CAD build for the part. Positions are in the model's coordinates, mm. Face numbers are marked on the shaded views. A direction names the side the tool comes from. Give positions to 0.01 mm unless a question says otherwise; leave off trailing zeros. Loops run counter-clockwise (first coordinate to the right, second up) from the corner with the lowest first, then second, coordinate; pieces in that order, holes last. Notation, with made-up numbers: M 80,56 L 121,56 A25 ccw 121,84 Z; hole C -0.75,9 d10. An arc over 180 degrees is marked long. Answer as CSV lines item,"result".
```python
from build123d import *

# Parameters (mm, degrees)
F0_R     = 26.67
F1_DEPTH = 3.175
F3_DEPTH = 25.4
F4_R     = 7.239
F5_DEPTH = 7.62
F7_DEPTH = 6.35
F8_R     = 2.159
F9_DEPTH = 25.4


with BuildPart() as f1:
    # F0 (on Front) → F1 (new body)
    with BuildSketch(Plane.XZ):
        Circle(F0_R)
    extrude(amount=F1_DEPTH)

    # F2 (on face) → F3 (cut)
    with BuildSketch(Plane.XZ.offset(3.175)):
        with BuildLine():
            Line((-21.59, 5.08), (-5.08, 5.08))
            Line((-5.08, 5.08), (-5.08, 21.59))
            ThreePointArc((-5.08, 21.59), (-5.221742, 22.173039), (-5.61533, 22.625934))
            ThreePointArc((-5.61533, 22.625934), (-16.90841, 16.90841), (-22.625934, 5.61533))
            ThreePointArc((-22.625934, 5.61533), (-22.173039, 5.221742), (-21.59, 5.08))
        make_face()
        with BuildLine():
            ThreePointArc((-21.59, -5.08), (-22.173039, -5.221742), (-22.625934, -5.61533))
            ThreePointArc((-22.625934, -5.61533), (-16.90841, -16.90841), (-5.61533, -22.625934))
            ThreePointArc((-5.61533, -22.625934), (-5.221742, -22.173039), (-5.08, -21.59))
            Line((-5.08, -21.59), (-5.08, -5.08))
            Line((-5.08, -5.08), (-21.59, -5.08))
        make_face()
        with BuildLine():
            ThreePointArc((5.08, -21.59), (5.221742, -22.173039), (5.61533, -22.625934))
            ThreePointArc((5.61533, -22.625934), (16.90841, -16.90841), (22.625934, -5.61533))
            ThreePointArc((22.625934, -5.61533), (22.173039, -5.221742), (21.59, -5.08))
            Line((21.59, -5.08), (5.08, -5.08))
            Line((5.08, -5.08), (5.08, -21.59))
        make_face()
        with BuildLine():
            ThreePointArc((21.59, 5.08), (22.173039, 5.221742), (22.625934, 5.61533))
            ThreePointArc((22.625934, 5.61533), (16.90841, 16.90841), (5.61533, 22.625934))
            ThreePointArc((5.61533, 22.625934), (5.221742, 22.173039), (5.08, 21.59))
            Line((5.08, 21.59), (5.08, 5.08))
            Line((5.08, 5.08), (21.59, 5.08))
        make_face()
    extrude(amount=-F3_DEPTH, mode=Mode.SUBTRACT)

    # F4 (on face) → F5 (join)
    with BuildSketch(Plane.XZ.offset(3.175)):
        Circle(F4_R)
    extrude(amount=F5_DEPTH)

    # F6 (on face) → F7 (cut)
    with BuildSketch(Plane.XZ.offset(10.795)):
        Polygon((3.519527, -6.096), (7.039054, 0), (3.519527, 6.096), (-3.519527, 6.096), (-7.039054, 0), (-3.519527, -6.096), align=None)
    extrude(amount=-F7_DEPTH, mode=Mode.SUBTRACT)

    # F8 (on face) → F9 (cut)
    with BuildSketch(Plane.XZ.offset(4.445)):
        Circle(F8_R)
    extrude(amount=-F9_DEPTH, mode=Mode.SUBTRACT)

    # F10 (on Top) → F11 (revolve, cut)
    with BuildSketch(Plane.XY):
        with BuildLine():
            Line((26.67, -2.667), (26.67, -0.508))
            ThreePointArc((26.67, -0.508), (25.743874, -1.5875), (26.67, -2.667))
        make_face()
    revolve(axis=Axis((0, -1.5875, 0), (0, -1, 0)), mode=Mode.SUBTRACT)


solid = f1.part
```
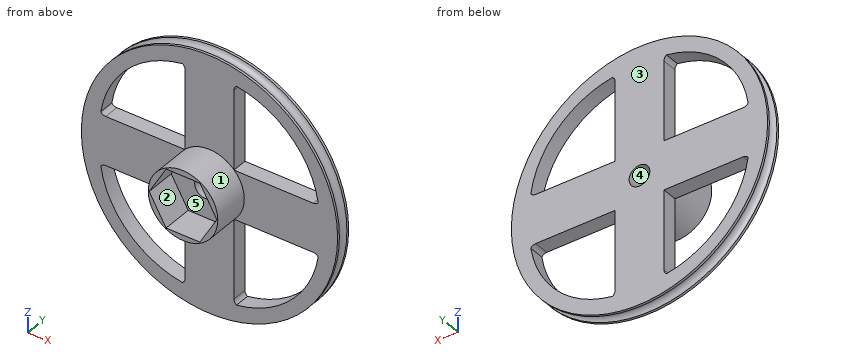
Q1. Cut at D-D (z = -13). Give the number of separate pieces and of enclosed holes in the cut face, and give its area (3 significant figures).
Solution:
separate pieces,"3"
enclosed holes,"0"
area,"49.9 mm²"
Q2. Pin check, flat tips, straight feed: P1, Ø3, axis at x = -0.5, y = -8, coming from the -Z side; P2, Ø1.9, axis at x = 1.5, y = -8, coming from the +Z side; P3, Ø2.5, axis at x = 0, z = 0, coming from the -Y side; P4, Ø3.5, axis at x = 13, y = -2.5, coming from the -Z side. Stop position of each tip, or through.
Solution:
P1,"stops at z = -7.24"
P2,"stops at z = 7.22"
P3,"passes through"
P4,"stops at z = -24.18"
Q3. Cut at C-C (y = -2). Write the cut outline in (x, z).
Solution:
outline,"C 0,0 d51.65; hole M -22.63,-5.62 A20.32 ccw -5.62,-22.63 A1.27 ccw -5.08,-21.59 L -5.08,-5.08 L -21.59,-5.08 A1.27 ccw Z; hole M -22.63,5.62 A1.27 ccw -21.59,5.08 L -5.08,5.08 L -5.08,21.59 A1.27 ccw -5.62,22.63 A20.32 ccw Z; hole C 0,0 d4.32; hole M 5.08,-21.59 A1.27 ccw 5.62,-22.63 A20.32 ccw 22.63,-5.62 A1.27 ccw 21.59,-5.08 L 5.08,-5.08 Z; hole M 5.08,5.08 L 21.59,5.08 A1.27 ccw 22.63,5.62 A20.32 ccw 5.62,22.63 A1.27 ccw 5.08,21.59 Z"
Q4. Which spindle directions (+Z, -Z, +X, -X, +Y, -Y) get a long thin tool onto all of the face, cutting with end or side? Do the marked faces 4 and 5. Say none if no direction does.
Solution:
face 4,"+Y, -Y"
face 5,"-Y"
Q5. Wall check: line 1 (Z direction, x = 0, y = -3.4); line 2 (Z direction, x = 0, y = -2.8); line 3 (Z direction, x = -18, y = -1.5). Give the ranges that are in metal, low to high. Write a range as [from, to].
Solution:
line 1,"z = [-7.24, -2.16], [2.16, 7.24]"
line 2,"z = [-26.67, -2.16], [2.16, 26.67]"
line 3,"z = [-18.41, -15.73], [-5.08, 5.08], [15.73, 18.41]"
Q6. Cut at A-A (y = -8). Write the cut outline in (x, z).
Solution:
outline,"C 0,0 d14.48; hole M -7.04,0 L -3.52,-6.1 L 3.52,-6.1 L 7.04,0 L 3.52,6.1 L -3.52,6.1 Z"
Q7. Mould opens along X. For the marked faces 1, 2 and 3 say: released by +X, released by -X, zero draft, split by the parting line, or undercut.
Solution:
face 1,"split by the parting line"
face 2,"undercut"
face 3,"zero draft"
Q8. Cut at B-B (x = 0). Write the cut outline in (y, z) (1 decimal), and give its area (3 significant figures).
Solution:
outline,"M -10.8,-7.2 L -3.2,-7.2 L -3.2,-26.7 L -2.7,-26.7 A1.1 cw -0.5,-26.7 L 0,-26.7 L 0,-2.2 L -4.4,-2.2 L -4.4,-6.1 L -10.8,-6.1 Z; M -10.8,6.1 L -4.4,6.1 L -4.4,2.2 L 0,2.2 L 0,26.7 L -0.5,26.7 A1.1 cw -2.7,26.7 L -3.2,26.7 L -3.2,7.2 L -10.8,7.2 Z"
area,"180 mm²"
